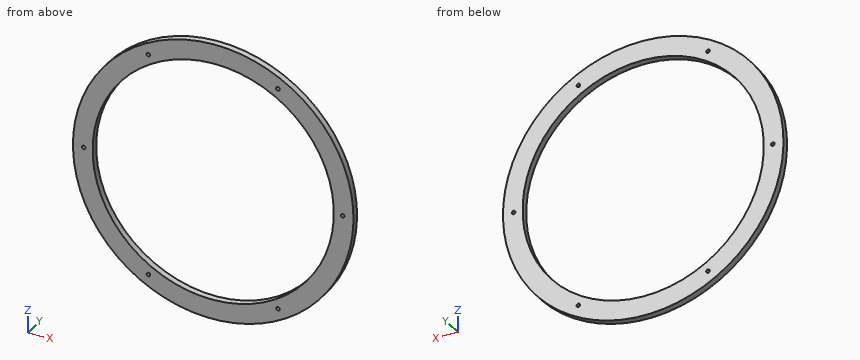
```python
from build123d import *

# Parameters (mm, degrees)
SKETCH1_R           = 392.5
SKETCH1_R_2         = 337.5
BOSS_EXTRUDE1_DEPTH = 9.5
SKETCH2_R           = 5
CUT_EXTRUDE1_DEPTH  = 556.40390708


with BuildPart() as part:
    # Sketch1 → Boss-Extrude1 (new, symmetric)
    with BuildSketch(Plane(origin=(0, 0, 0), x_dir=(1, 0, 0), z_dir=(0, 1, 0))):
        with Locations(Location((0, 0, 0), (0, 0, 270))):
            Circle(SKETCH1_R)
        with Locations(Location((0, 0, 0), (0, 0, 270))):
            Circle(SKETCH1_R_2, mode=Mode.SUBTRACT)
    extrude(amount=BOSS_EXTRUDE1_DEPTH, both=True)

    # Sketch2 → Cut-Extrude1 (cut, through all)
    with BuildSketch(Plane(origin=(0, 9.5, 0), x_dir=(1, 0, 0), z_dir=(0, 1, 0))):
        with Locations(Location((181.25, 313.934208872, 0), (0, 0, 270))):
            Circle(SKETCH2_R)
        with Locations(Location((362.5, 0, 0), (0, 0, 270))):
            Circle(SKETCH2_R)
        with Locations(Location((181.25, -313.934208872, 0), (0, 0, 270))):
            Circle(SKETCH2_R)
        with Locations(Location((-181.25, -313.934208872, 0), (0, 0, 270))):
            Circle(SKETCH2_R)
        with Locations(Location((-362.5, 0, 0), (0, 0, 270))):
            Circle(SKETCH2_R)
        with Locations(Location((-181.25, 313.934208872, 0), (0, 0, 270))):
            Circle(SKETCH2_R)
    extrude(amount=-CUT_EXTRUDE1_DEPTH, mode=Mode.SUBTRACT)


solid = part.part
```
Read the model definition and answer for the solid it produces. Units are mm, in the model's axes. Give positions to 0.01 mm unless a question says otherwise; leave off trailing zeros. Order: outer loops, then holes, each group sorted by start corner. A loop starts at its lowest first (then second) coordinate and runs counter-clockwise, first axis right, second up. Notation, with made-up numbers: (-23.75, -38) -> (21.25, -38) arc R18 ccw to (21.25, -19) -> close; hole circle Ø7 at (85.5, 87). An arc over 180 degrees is marked (long way). Write item = value, one per line.
1. A cutting plane is placed at A-A, the plane x = 0. Write down the section's boundary in (y, z), and give its area (3 significant figures).
Numbers:
outline = (-9.5, -392.5) -> (9.5, -392.5) -> (9.5, -337.5) -> (-9.5, -337.5) -> close; (-9.5, 337.5) -> (9.5, 337.5) -> (9.5, 392.5) -> (-9.5, 392.5) -> close
area = 2,090 mm²
2. A cutting plane is placed at C-C, the plane z = -238. Write down the section's boundary in (x, y).
Numbers:
outline = (-312.11, -9.5) -> (-239.3, -9.5) -> (-239.3, 9.5) -> (-312.11, 9.5) -> close; (239.3, -9.5) -> (312.11, -9.5) -> (312.11, 9.5) -> (239.3, 9.5) -> close
3. Straight lines are drawn through the part: line 1 along X through (y, z) = (-5.25, 0); line 2 along Z through (x, y) = (-32.5, 4.5); line 3 along X through (y, z) = (-2.25, -104.5). For each, find the intervals that lie inside material, in ascending order.
Numbers:
line_1 = -392.5 to -367.5, -357.5 to -337.5, 337.5 to 357.5, 367.5 to 392.5
line_2 = -391.15 to -335.93, 335.93 to 391.15
line_3 = -378.33 to -320.91, 320.91 to 378.33
4. A cutting plane is placed at B-B, the plane y = -0.25. Write down the section's boundary in (x, z), and give its area (3 significant figures).
Numbers:
outline = circle Ø785 at (0, 0); hole circle Ø10 at (-362.5, 0); hole circle Ø675 at (0, 0); hole circle Ø10 at (-181.25, -313.93); hole circle Ø10 at (-181.25, 313.93); hole circle Ø10 at (181.25, -313.93); hole circle Ø10 at (181.25, 313.93); hole circle Ø10 at (362.5, 0)
area = 126,000 mm²
5. Given pin 1 (8 mm diameter, centred on y = -7, z = -166.5, fed in from +X); pin 2 (9 mm diameter, centred on x = 362.5, z = 0, fed in from -Y); pin 3 (2 mm diameter, centred on x = 219.5, y = 0, fed in from -Z); pin 4 (3 mm diameter, centred on y = 4, z = -108.5, fed in from -X), each flat-ended and moving along its own axis, determine where each tip first touches the part or whether it passes through.
Numbers:
pin_1 = 357.28
pin_2 = through
pin_3 = -326.06
pin_4 = -377.63
